Source: CAD feature listing. Evaluate the final solid. Frame: model axes, mm. Face numbers are marked on the shaded views. A direction names the side the tool comes from. Round coordinates to 2 decimals unless told otherwise and drop trailing zeros. Loops run counter-clockwise (first coordinate to the right, second up) from the corner with the lowest first, then second, coordinate; pieces in that order, holes last. Notation, with made-up numbers: (-30, 22.5) -> (-24, 22.5) arc R26 ccw to (-24, 51.5) -> close; hole circle Ø10 at (-30, 87). An arc over 180 degrees is marked (long way). Put each result on its own line as item: value. Start each with the question number.
1. Cut plane B-B (y = -0.5). Return the cut outline in (x, z).
2. Contact query for flat-ended pins moving along their axis: pin 1 (1 mm diameter, centred on y = -1, z = -20, fed in from +X); pin 2 (4 mm diameter, centred on x = 18.5, z = -15, fed in from +Y); pin 3 (4 mm diameter, centred on x = 17.5, z = -17.5, fed in from +Y). Output: stop coordinate, or through.
3. Cut plane A-A (x = 17.5). Return the cut outline in (y, z) (1 decimal), then the cut area to 3 significant figures.
4. Material intervals for L1, parallel to Z at x = 17.5, y = -1.75; L2, parallel to X at y = -0.7, z = -17.5; L3, parallel to Z at x = 17.5, y = -0.7, sorted ascending.
5. Set-up query: the marked faces 1 and 2. Return all of +Z, -Z, +X, -X, +Y, -Y with unobstructed straight access to the full face (end or side cutting, diameter ignored); none if empty.
6. Cut plane D-D (z = -10.5). Return the cut outline in (x, y) (3 decimals).
7. Cut plane C-C (z = -17.5). Return the cut outline in (x, y) (1 decimal).
Autodesk Inventor part; units mm, degrees
ref_plane "YZ Plane" through (0, 0, 0) normal (1, 0, 0) x (0, 1, 0)
ref_plane "XZ Plane" through (0, 0, 0) normal (0, 1, 0) x (-1, 0, 0)
ref_plane "XY Plane" through (0, 0, 0) normal (0, 0, 1) x (1, 0, 0)
sketch "Sketch1" plane through (0, 0, 0) normal (0, 1, 0) x (-1, 0, 0)
  line L0 (0, -2) -> (0, -38)
  line L1 (-2, 0) -> (-38, 0)
  line L2 (-40, -2) -> (-40, -8)
  line L3 (-38, -10) -> (-27, -10)
  line L4 (-10, -27) -> (-10, -38)
  line L5 (-8, -40) -> (-2, -40)
  line L6 (-12, -25) -> (-23, -25)
  line L7 (-25, -23) -> (-25, -12)
  arc A0 (-10, -27) -> (-12, -25) centre (-12, -27) ccw
  arc A1 (-25, -23) -> (-23, -25) centre (-23, -23) ccw
  arc A2 (-25, -12) -> (-27, -10) centre (-27, -12) ccw
  arc A3 (-10, -38) -> (-8, -40) centre (-8, -38) ccw
  arc A4 (-40, -8) -> (-38, -10) centre (-38, -8) ccw
  arc A5 (-38, 0) -> (-40, -2) centre (-38, -2) ccw
  arc A6 (0, -2) -> (-2, 0) centre (-2, -2) ccw
  arc A7 (-2, -40) -> (0, -38) centre (-2, -38) ccw
  line L8 (-27, -10) -> (-12, -10)
  line L9 (-10, -27) -> (-10, -12)
  arc A8 (-10, -12) -> (-12, -10) centre (-12, -12) ccw
  point P0 (0, 0)
  point P1 (0, -40)
  point P2 (-40, 0)
  point P3 (-40, -10)
  point P4 (-10, -10)
  point P5 (-10, -40)
  point P6 (-10, -25)
  point P7 (-25, -25)
  point P8 (-25, -10)
  point P9 (-17.5, -17.5)
  dimension "d0" = 40
  dimension "d2" = 10
  dimension "d8" = 15
  dimension "d9" = 15
  dimension "d11" = 10
  dimension "d12" = 40
  dimension "d13" = 2
  dimension "d14" = 2
extrude "Extrusion1" add sketch "Sketch1" along normal blind 1.175 contours L0 A7 L5 A3 L4 L9 A8 L8 L3 A4 L2 A5 L1 A6
extrude "Extrusion2" add sketch "Sketch1" against normal blind 2
hole "Hole1" at (17.5, 0, -17.5) direction (0, -1, 0) diameter 2.459 depth 8.8 tip angle 118 counterbore diameter 6 counterbore depth 1
properties part number "Standoff_Corner"
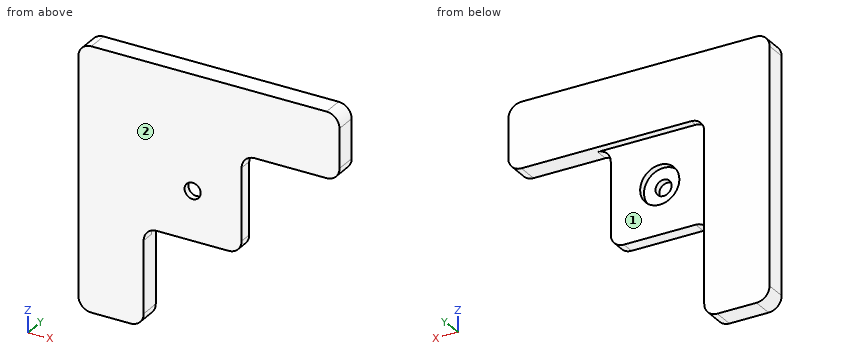
Solution:
1. outline: (0, -38) arc R2 ccw to (2, -40) -> (8, -40) arc R2 ccw to (10, -38) -> (10, -27) arc R2 cw to (12, -25) -> (23, -25) arc R2 ccw to (25, -23) -> (25, -12) arc R2 cw to (27, -10) -> (38, -10) arc R2 ccw to (40, -8) -> (40, -2) arc R2 ccw to (38, 0) -> (2, 0) arc R2 ccw to (0, -2) -> close; hole circle Ø6 at (17.5, -17.5)
2. pin 1: stops at x = 25
2. pin 2: stops at y = 0
2. pin 3: stops at y = -1
3. outline: (-2, -25) -> (0, -25) -> (0, -20.5) -> (-1, -20.5) -> (-1, -18.7) -> (-2, -18.7) -> close; (-2, -16.3) -> (-1, -16.3) -> (-1, -14.5) -> (0, -14.5) -> (0, -10) -> (1.2, -10) -> (1.2, 0) -> (-2, 0) -> close
3. area: 53.3 mm^2
4. L1: z = -25 to -18.73, -16.27 to 0
4. L2: x = 0 to 14.5, 20.5 to 25
4. L3: z = -25 to -20.5, -14.5 to 0
5. face 1: -Z, +X, +Y
5. face 2: +Z, -Z, +X, -X, -Y
6. outline: (0, -2) -> (25.677, -2) -> (25.677, 0) -> (10.677, 0) -> (10.677, 1.175) -> (0, 1.175) -> close
7. outline: (0, -2) -> (16.3, -2) -> (16.3, -1) -> (14.5, -1) -> (14.5, 0) -> (10, 0) -> (10, 1.2) -> (0, 1.2) -> close; (18.7, -2) -> (25, -2) -> (25, 0) -> (20.5, 0) -> (20.5, -1) -> (18.7, -1) -> close
